from build123d import *

# Parameters (mm, degrees)
SKETCH_W     = 130
SKETCH_H     = 68
PAD_DEPTH    = 1
SKETCH001_W  = 100
SKETCH001_H  = 1
PAD001_DEPTH = 3
SKETCH002_W  = 100
SKETCH002_H  = 1
PAD002_DEPTH = 3
PAD003_DEPTH = 3
SKETCH004_W  = 100
SKETCH004_H  = 1
PAD004_DEPTH = 28
SKETCH005_W  = 100
SKETCH005_H  = 1
PAD005_DEPTH = 28
PAD006_DEPTH = 28
SKETCH007_W  = 100
SKETCH007_H  = 2.7
PAD007_DEPTH = 25


with BuildPart() as part:
    # Sketch → Pad (new body)
    with BuildSketch(Plane.XY):
        with Locations((65, 34)):
            Rectangle(SKETCH_W, SKETCH_H)
    extrude(amount=-PAD_DEPTH)

    # Sketch001 → Pad001 (join)
    with BuildSketch(Plane.XY):
        with Locations((54, 7.5)):
            Rectangle(SKETCH001_W, SKETCH001_H)
    extrude(amount=PAD001_DEPTH)

    # Sketch002 → Pad002 (join)
    with BuildSketch(Plane.XY):
        with Locations((54, 11.2)):
            Rectangle(SKETCH002_W, SKETCH002_H)
    extrude(amount=PAD002_DEPTH)

    # Sketch003 → Pad003 (join)
    with BuildSketch(Plane.XY):
        Polygon((104, 10.7), (114, 19), (112.795181, 19), (104, 11.7), align=None)
        Polygon((104, 8), (114, 3.7), (111.674419, 3.7), (104, 7), align=None)
    extrude(amount=PAD003_DEPTH)

    # Sketch004 → Pad004 (join)
    with BuildSketch(Plane.XY):
        with Locations((54, 56.8)):
            Rectangle(SKETCH004_W, SKETCH004_H)
    extrude(amount=PAD004_DEPTH)

    # Sketch005 → Pad005 (join)
    with BuildSketch(Plane.XY):
        with Locations((54, 60.5)):
            Rectangle(SKETCH005_W, SKETCH005_H)
    extrude(amount=PAD005_DEPTH)

    # Sketch006 → Pad006 (join)
    with BuildSketch(Plane.XY):
        Polygon((104, 61), (112, 65), (114, 65), (104, 60), align=None)
        Polygon((104, 57.3), (109, 55), (106.826087, 55), (104, 56.3), align=None)
    extrude(amount=PAD006_DEPTH)

    # Sketch007 → Pad007 (join)
    with BuildSketch(Plane.XY):
        with Locations((54, 58.65)):
            Rectangle(SKETCH007_W, SKETCH007_H)
    extrude(amount=PAD007_DEPTH)


solid = part.part
Geometry: final body of the model. Coordinates: model frame, mm. A direction names the side the tool comes from. Give positions to 0.01 mm unless a question says otherwise; leave off trailing zeros. Write each loop counter-clockwise with the first axis right and the second up, starting at its lowest first coordinate (ties: lowest second). Pieces come first, ordered by that corner, then holes. Notation, with made-up numbers: (-28, 72.5) - (-17, 72.5) arc R11 cw to (-17, 90.5) - close; hole circle Ø5 at (-17, 59.25). An arc over 180 degrees is marked (long way). Return JSON: item names as keys, results as strings. Group by question number.
1) Section C-C on y = 45. Return the cut outline in (x, z), plus the area to 3 significant figures.
2) Mould query, pull axis Y, two halves, no side actions, for faces 5 (the flat face through (53, 61, 14)), 6 (the flat face through (108.46, 15.4, 1.48)), 7 (the flat face through (53, 10.7, 1)), 8 (the flat face through (56, 57, 28)). Classes: released by +Y, released by -Y, zero draft, split by the parting line, or undercut.
3) Section A-A on z = 1.75. Return the cut outline in (x, y), plus the area to 3 significant figures.
4) First-contact query: P1, Ø6, axis at x = 41.5, y = 53.5, coming from the +Z side; P2, Ø12, axis at x = 40.5, z = 14, coming from the +Y side; P3, Ø1.6, axis at x = 113, z = 14, coming from the +Y side; P4, Ø0.8, axis at y = 58.5, z = 18.5, coming from the +X side. Flat tips, straight axial feed; report the tip coordinate or a pass-through.
5) Set-up query: faces 1 (the flat face through (53, 59, 25)), 2 (the flat face through (104, 59, 12)), 3 (the flat face through (108, 63, 14)), 4 (the flat face through (53, 11.7, 1)). Return all of +Z, -Z, +X, -X, +Y, -Y with unobstructed straight access to the full face (end or side cutting, diameter ignored); none if empty.
6) Line query: line 1 (Y direction, x = 42.5, z = 1.5); line 2 (Z direction, x = 27, y = 44); line 3 (Y direction, x = 75.5, z = 25.5). Output: solid intervals per line, ascending.
7) Section B-B on x = 23. Return the cut outline in (y, z).
8) Section D-D on z = 8. Return the cut outline in (x, y).
Filled in:
{
 "1": {"outline": "(0, -1) - (130, -1) - (130, 0) - (0, 0) - close", "area": "130 mm^2"},
 "2": {"face 5": "released by +Y", "face 6": "undercut", "face 7": "undercut", "face 8": "zero draft"},
 "3": {"outline": "(4, 7) - (104, 7) - (111.67, 3.7) - (114, 3.7) - (104, 8) - (4, 8) - close; (4, 10.7) - (104, 10.7) - (114, 19) - (112.8, 19) - (104, 11.7) - (4, 11.7) - close; (4, 56.3) - (104, 56.3) - (106.83, 55) - (109, 55) - (104, 57.3) - (104, 60) - (114, 65) - (112, 65) - (104, 61) - (4, 61) - close", "area": "701 mm^2"},
 "4": {"P1": "stops at z = 28", "P2": "stops at y = 61", "P3": "stops at y = 65", "P4": "stops at x = 104"},
 "5": {"face 1": "+Z, +X, -X", "face 2": "+Z, +X", "face 3": "+Z, -X, +Y", "face 4": "+Z, -X"},
 "6": {"line 1": "y = 7 to 8, 10.7 to 11.7, 56.3 to 61", "line 2": "z = -1 to 0", "line 3": "y = 56.3 to 57.3, 60 to 61"},
 "7": {"outline": "(0, -1) - (68, -1) - (68, 0) - (61, 0) - (61, 28) - (60, 28) - (60, 25) - (57.3, 25) - (57.3, 28) - (56.3, 28) - (56.3, 0) - (11.7, 0) - (11.7, 3) - (10.7, 3) - (10.7, 0) - (8, 0) - (8, 3) - (7, 3) - (7, 0) - (0, 0) - close"},
 "8": {"outline": "(4, 56.3) - (104, 56.3) - (106.83, 55) - (109, 55) - (104, 57.3) - (104, 60) - (114, 65) - (112, 65) - (104, 61) - (4, 61) - close"}
}
